```python
from build123d import *

# Parameters (mm, degrees)
SKETCH1_R           = 15
BOSS_EXTRUDE1_DEPTH = 200
BOSS_EXTRUDE2_DEPTH = 10
BOSS_EXTRUDE3_DEPTH = 10
CHAMFER1_SIZE       = 4


with BuildPart() as part:
    # Sketch1 → Boss-Extrude1 (new body)
    with BuildSketch(Plane.XY):
        Circle(SKETCH1_R)
    extrude(amount=BOSS_EXTRUDE1_DEPTH)

    # Sketch3 → Boss-Extrude2 (add)
    with BuildSketch(Plane(origin=(0, 0, 0), x_dir=(-1, 0, 0), z_dir=(0, 0, -1))):
        Polygon((18.338660343, 0), (9.169330171, 15.881745728), (-9.169330171, 15.881745728), (-18.338660343, 0), (-9.169330171, -15.881745728), (9.169330171, -15.881745728), align=None)
    extrude(amount=BOSS_EXTRUDE2_DEPTH)

    # Sketch2 → Boss-Extrude3 (add)
    with BuildSketch(Plane.XY.offset(200)):
        Polygon((18.338660343, 0), (9.169330171, 15.881745728), (-9.169330171, 15.881745728), (-18.338660343, 0), (-9.169330171, -15.881745728), (9.169330171, -15.881745728), align=None)
    extrude(amount=BOSS_EXTRUDE3_DEPTH)

    # Chamfer1
    chamfer1_edges = [part.edges().sort_by_distance(p)[0] for p in [
        (13.753995257, -7.940872864, 210),
        (13.753995257, 7.940872864, 210),
        (0, 15.881745728, 210),
        (-13.753995257, 7.940872864, 210),
        (-13.753995257, -7.940872864, 210),
        (0, -15.881745728, 210),
        (-13.753995257, -7.940872864, -10),
        (-13.753995257, 7.940872864, -10),
        (0, 15.881745728, -10),
        (13.753995257, 7.940872864, -10),
        (13.753995257, -7.940872864, -10),
        (0, -15.881745728, -10),
    ]]
    chamfer(chamfer1_edges, length=CHAMFER1_SIZE)


solid = part.part
```
The model under review builds one solid part; all positions refer to its coordinate system, in mm. Round coordinates to 2 decimals unless told otherwise and drop trailing zeros. Order: outer loops, then holes, each group sorted by start corner. A loop starts at its lowest first (then second) coordinate and runs counter-clockwise, first axis right, second up. Notation, with made-up numbers: (-35.75, 60.5) - (16.25, 60.5) arc R19 ccw to (16.25, 70.5) - close; hole circle Ø7 at (-35, 41.25). An arc over 180 degrees is marked (long way). Answer in a Markdown table with one row per item.
(1) Take a section at A-A on x = 0. Write out the cut boundary in (y, z), plus the area to 3 significant figures.
Result set:
| item | result |
|---|---|
| outline | (-15.88, -6) - (-11.88, -10) - (11.88, -10) - (15.88, -6) - (15.88, 0) - (15, 0) - (15, 200) - (15.88, 200) - (15.88, 206) - (11.88, 210) - (-11.88, 210) - (-15.88, 206) - (-15.88, 200) - (-15, 200) - (-15, 0) - (-15.88, 0) - close |
| area | 6,600 mm2 |
(2) Take a section at B-B on y = 4. Write out the cut boundary in (x, z).
Result set:
| item | result |
|---|---|
| outline | (-16.03, -6) - (-11.41, -10) - (11.41, -10) - (16.03, -6) - (16.03, 0) - (14.46, 0) - (14.46, 200) - (16.03, 200) - (16.03, 206) - (11.41, 210) - (-11.41, 210) - (-16.03, 206) - (-16.03, 200) - (-14.46, 200) - (-14.46, 0) - (-16.03, 0) - close |
(3) For line 1 (Y direction, x = 6, z = 186.5); line 2 (Z direction, x = -10.5, y = -12.5); line 3 (X direction, y = 9.5, z = 101.5), list the stretches that pass through material, from the lowest coordinate up. Write a range as from..to.
Result set:
| item | result |
|---|---|
| line 1 | y = -13.75..13.75 |
| line 2 | z = -6.54..0, 200..206.54 |
| line 3 | x = -11.61..11.61 |
(4) Clearance check with flat-ended pins moving along their axes: P1, Ø2, axis at x = -12, y = -9, coming from the +Z side; P2, Ø5, axis at x = -12, z = 41, coming from the -Y side; P3, Ø3, axis at x = -10, z = 184, coming from the -Y side. State where each tip first meets the part, or that it passes through.
Result set:
| item | result |
|---|---|
| P1 | stops at z = 207.99 |
| P2 | stops at y = -11.61 |
| P3 | stops at y = -12.36 |
(5) Take a section at C-C on z = 170.5. Write out the cut boundary in (x, y), plus the area to 3 significant figures.
Result set:
| item | result |
|---|---|
| outline | circle Ø30 at (0, 0) |
| area | 707 mm2 |
